The figure shows three views and two pictorial views of one solid part (mm, origin at its lowest corner). Answer the questions. A direction names the side the tool comes from. Round coordinates to 2 decimals unless told otherwise and drop trailing zeros. Order: outer loops, then holes, each group sorted by start corner. A loop starts at its lowest first (then second) coordinate and runs counter-clockwise, first axis right, second up. Notation, with made-up numbers: (28.25, 51.5) -> (74.25, 51.5) arc R16 cw to (74.25, 73.5) -> close; hole circle Ø2 at (-33, 46). An arc over 180 degrees is marked (long way). Answer as a JSON object with one key per item and string values. Group by question number.
Item 1: Given P1, Ø3, axis at y = 1.5, z = 9, coming from the +X side; P2, Ø3, axis at y = 1.5, z = 6, coming from the -X side; P3, Ø1, axis at y = 3.5, z = 9.5, coming from the +X side, each flat-ended and moving along its own axis, determine where each tip first touches the part or whether it passes through.
Item 2: Section A-A, the plane x = 17 is taken. Write down the section's boundary in (y, z), plus the area to 3 significant figures.
Item 3: Section C-C, the plane x = 4 is taken. Write down the section's boundary in (y, z).
Item 4: Consider probe 1 along Z at (x, y) = (2, 1.5); probe 2 along Y at (x, z) = (4, 2.5); probe 3 along X at (y, z) = (6.4, 6). Determine where each line is inside the solid, lowest interval first. Write a range as from..to.
Item 5: Section D-D, the plane y = 3.5 is taken. Write down the section's boundary in (x, z).
Item 6: For the marked faces 5, 6, 7, 8 and 9, determine the directions among +Z, -Z, +X, -X, +Y, -Y from which every point of the face is accessible in a straight line to the end or side of a thin tool.
Item 7: Section B-B, the plane z = 6 is taken. Write down the section's boundary in (x, y), plus the area to 3 significant figures.
Item 8: The mould has two halves that part along Y. Classify the marked faces 1, 2, 3 and 4: pulls with the +Y half, pulls with the -Y half, needs draft (parallel to the pull), parting line crosses it, or undercut.
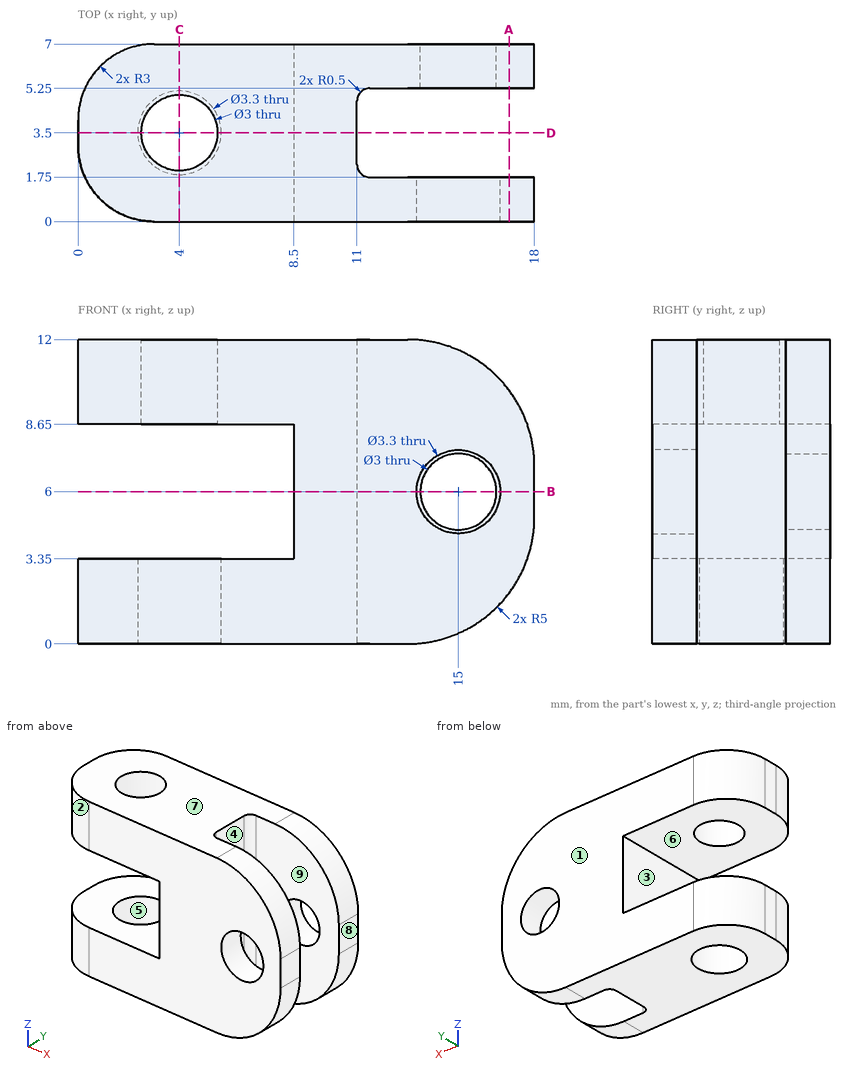
Values found:
{
 "1": {"P1": "x = 17.97", "P2": "x = 8.5", "P3": "x = 11"},
 "2": {"outline": "(0, 2) -> (1.75, 2) -> (1.75, 10) -> (0, 10) -> close; (5.25, 2) -> (7, 2) -> (7, 10) -> (5.25, 10) -> close", "area": "28.0 mm2"},
 "3": {"outline": "(0, 0) -> (1.85, 0) -> (1.85, 3.35) -> (0, 3.35) -> close; (0, 8.65) -> (2, 8.65) -> (2, 12) -> (0, 12) -> close; (5, 8.65) -> (7, 8.65) -> (7, 12) -> (5, 12) -> close; (5.15, 0) -> (7, 0) -> (7, 3.35) -> (5.15, 3.35) -> close"},
 "4": {"probe 1": "0..3.35, 8.65..12", "probe 2": "0..1.85, 5.15..7", "probe 3": "8.5..13.5, 16.5..18"},
 "5": {"outline": "(0, 0) -> (2.35, 0) -> (2.35, 3.35) -> (0, 3.35) -> close; (0, 8.65) -> (2.5, 8.65) -> (2.5, 12) -> (0, 12) -> close; (5.5, 8.65) -> (8.5, 8.65) -> (8.5, 3.35) -> (5.65, 3.35) -> (5.65, 0) -> (11, 0) -> (11, 12) -> (5.5, 12) -> close"},
 "6": {"face 5": "-Z", "face 6": "-X, +Y, -Y", "face 7": "+Z, +X, -X, +Y, -Y", "face 8": "+Z, -Z, +X, +Y, -Y", "face 9": "+Z, -Z, +X"},
 "7": {"outline": "(8.5, 0) -> (13.35, 0) -> (13.35, 1.75) -> (11.5, 1.75) arc R0.5 cw to (11, 2.25) -> (11, 4.75) arc R0.5 cw to (11.5, 5.25) -> (13.5, 5.25) -> (13.5, 7) -> (8.5, 7) -> close; (16.5, 5.25) -> (18, 5.25) -> (18, 7) -> (16.5, 7) -> close; (16.65, 0) -> (18, 0) -> (18, 1.75) -> (16.65, 1.75) -> close", "area": "31.1 mm2"},
 "8": {"face 1": "pulls with the +Y half", "face 2": "pulls with the -Y half", "face 3": "needs draft", "face 4": "undercut"}
}
